Can you work these out from the model? Positions are in its coordinate system, mm. A direction names the side the tool comes from. Round coordinates to 2 decimals unless told otherwise and drop trailing zeros. Loops run counter-clockwise (first coordinate to the right, second up) from the corner with the lowest first, then second, coordinate; pieces in that order, holes last.
(1) Thinking about a two-plate mould opening in Y: for faces 1 (the face through (1.283, 205.966, -3.858)), 2 (the face through (8, 368, 3)), 3 (the face through (1.283, 205.966, 10.142)), 4 (the face through (1, 181, 9.156)), which applies, released by +Y, released by -Y, zero draft, split by the parting line, or undercut?
(2) Which directions (+Z, -Z, +X, -X, +Y, -Y) give clear straight access to the entire face, cutting with the end or side of a thin tool? Please do faces 5 (the face through (8.762, 181, 3)), 6 (the face through (1, 181, -2.844)).
(3) I want a section at B-B on y = 276. Write out the boundary of the cut face in (x, z).
(4) I want a section at A-A on y = 202. Write out the boundary of the cut face in (x, z).
(5) If I drill on line 1 along Z through (x, y) = (-0.75, 283.5); line 2 along X through (y, z) = (86.5, 7); line 3 along Y through (x, z) = (-5.5, 2), over which ranges is the centre line in solid material (lowest first)?
(6) Will this pin go through, and if not, where does the flat tip stop? pin 1 Ø4.5 at (x, y) = (3.75, 358.56) entering from +Z.
from build123d import *

# Parameters (mm, degrees)
SKETCH1_W           = 16
SKETCH1_H           = 16
SKETCH1_W_2         = 12
SKETCH1_H_2         = 12
BOSS_EXTRUDE1_DEPTH = 368
FILLET1_R           = 1
SKETCH2_R           = 1.75
CUT_EXTRUDE1_DEPTH  = 16
SKETCH3_R           = 4
CUT_EXTRUDE2_DEPTH  = 16
SKETCH4_R           = 2.5
CUT_EXTRUDE3_DEPTH  = 20


with BuildPart() as part:
    # Sketch1 → Boss-Extrude1 (new body)
    with BuildSketch(Plane(origin=(0, 0, 0), x_dir=(1, 0, 0), z_dir=(0, 1, 0))):
        with Locations((0.761904762, -3.156462585)):
            Rectangle(SKETCH1_W, SKETCH1_H)
        with Locations((0.761904762, -3.156462585)):
            Rectangle(SKETCH1_W_2, SKETCH1_H_2, mode=Mode.SUBTRACT)
    extrude(amount=BOSS_EXTRUDE1_DEPTH)

    # Fillet1
    fillet1_edges = [part.edges().sort_by_distance(p)[0] for p in [
        (-7.238095238, 184, -4.843537415),
        (8.761904762, 184, -4.843537415),
        (8.761904762, 184, 11.156462585),
        (-7.238095238, 184, 11.156462585),
    ]]
    fillet(fillet1_edges, radius=FILLET1_R)

    # Sketch2 → Cut-Extrude1 (cut)
    with BuildSketch(Plane.ZY.offset(7.238095238)):
        with Locations((3.156462585, 5.25)):
            Circle(SKETCH2_R)
        with Locations((3.156462585, 20.25)):
            Circle(SKETCH2_R)
        with Locations((3.156462585, 35.25)):
            Circle(SKETCH2_R)
    extrude(amount=-CUT_EXTRUDE1_DEPTH, mode=Mode.SUBTRACT)

    # Sketch3 → Cut-Extrude2 (cut)
    with BuildSketch(Plane(origin=(0, 0, -4.843537415), x_dir=(-1, 0, 0), z_dir=(0, 0, -1))):
        with Locations((-0.761904762, 202)):
            Circle(SKETCH3_R)
    extrude(amount=-CUT_EXTRUDE2_DEPTH, mode=Mode.SUBTRACT)

    # Sketch4 → Cut-Extrude3 (cut)
    with BuildSketch(Plane.XY.offset(11.156462585)):
        with Locations((-2.232226364, 353.25267067)):
            Circle(SKETCH4_R)
        with Locations((3.753864965, 358.559902585)):
            Circle(SKETCH4_R)
    extrude(amount=-CUT_EXTRUDE3_DEPTH, mode=Mode.SUBTRACT)


solid = part.part
Filled sheet:
1. face 1: undercut
1. face 2: released by +Y
1. face 3: undercut
1. face 4: zero draft
2. face 5: +Z, -Z, +X, +Y, -Y
2. face 6: +Y, -Y
3. outline: (-7.24, -3.84) arc R1 ccw to (-6.24, -4.84) - (7.76, -4.84) arc R1 ccw to (8.76, -3.84) - (8.76, 10.16) arc R1 ccw to (7.76, 11.16) - (-6.24, 11.16) arc R1 ccw to (-7.24, 10.16) - close; hole (-5.24, -2.84) - (6.76, -2.84) - (6.76, 9.16) - (-5.24, 9.16) - close
4. outline: (-7.24, -3.84) arc R1 ccw to (-6.24, -4.84) - (-3.24, -4.84) - (-3.24, -2.84) - (-5.24, -2.84) - (-5.24, 9.16) - (-3.24, 9.16) - (-3.24, 11.16) - (-6.24, 11.16) arc R1 ccw to (-7.24, 10.16) - close; (4.76, -4.84) - (7.76, -4.84) arc R1 ccw to (8.76, -3.84) - (8.76, 10.16) arc R1 ccw to (7.76, 11.16) - (4.76, 11.16) - (4.76, 9.16) - (6.76, 9.16) - (6.76, -2.84) - (4.76, -2.84) - close
5. line 1: z = -4.84 to -2.84, 9.16 to 11.16
5. line 2: x = -7.24 to -5.24, 6.76 to 8.76
5. line 3: y = 0 to 3.94, 6.56 to 18.94, 21.56 to 33.94, 36.56 to 368
6. pin 1: passes through
